Could you check a few things on this model? Use its own coordinates, in mm. A direction names the side the tool comes from. Coordinates: 2 decimals unless noted, no trailing zeros. Loops run counter-clockwise (first coordinate to the right, second up) from the corner with the lowest first, then second, coordinate; pieces in that order, holes last. Notation, with made-up numbers: (58, -29) -> (63, -29) arc R26 cw to (63, 8) -> close; hole circle Ø1 at (65, 71). An arc over 180 degrees is marked (long way). One line per question, with ' | ' between items.
from build123d import *

# Parameters (mm, degrees)
F0_R     = 2
F0_R_2   = 5
F1_DEPTH = 12
F2_R     = 2
F3_DEPTH = 25
F4_R     = 4.99999


# Not quite as in the source:
# - a fillet or chamfer is up to 0.001 mm smaller than in the source, because OpenCascade refuses the exact size


with BuildPart() as f1:
    # F0 (on Top) → F1 (new body)
    with BuildSketch(Plane.XY):
        with BuildLine():
            Line((-35.0000017881, -70), (35.0000017881, -70))
            ThreePointArc((35.0000017881, -70), (42.0710696, -67.0710678119), (45.0000017881, -60))
            Line((45.0000017881, -60), (45.0000017881, 70))
            Line((45.0000017881, 70), (-45.0000017881, 70))
            Line((-45.0000017881, 70), (-45.0000017881, -60))
            ThreePointArc((-45.0000017881, -60), (-42.0710696, -67.0710678119), (-35.0000017881, -70))
        make_face()
        with Locations((0, -30)):
            Circle(F0_R, mode=Mode.SUBTRACT)
        with Locations((0, 30)):
            Circle(F0_R, mode=Mode.SUBTRACT)
        with Locations((-35.0000017881, 60)):
            Circle(F0_R_2, mode=Mode.SUBTRACT)
        with Locations((0, 60)):
            Circle(F0_R_2, mode=Mode.SUBTRACT)
        with Locations((35.0000017881, 60)):
            Circle(F0_R_2, mode=Mode.SUBTRACT)
    extrude(amount=F1_DEPTH)

    # F2 (on face) → F3 (cut)
    with BuildSketch(Plane(origin=(0, 70, 0), x_dir=(-1, 0, 0), z_dir=(0, 1, 0))):
        with Locations((0, 6)):
            Circle(F2_R)
        with Locations((35.0000017881, 6)):
            Circle(F2_R)
        with Locations((-35.0000017881, 6)):
            Circle(F2_R)
    extrude(amount=-F3_DEPTH, mode=Mode.SUBTRACT)

    # F4 (radius 5 in the source; OpenCascade refuses exactly that, so slightly less here)
    f4_edges = [f1.edges().sort_by_distance(p)[0] for p in [
        (45.000002, 5, 0),
    ]]
    fillet(f4_edges, radius=F4_R)


solid = f1.part
1) If we section it at C-C on y = 60: Give the number of separate pieces and of enclosed holes in the cut face, and give its area (3 significant figures).
Data:
separate pieces: 4 | enclosed holes: 0 | area: 709 mm²
2) I'm going to push a flat-ended pin straight in: pin 1 Ø1.2 at (x, z) = (34.5, 6) entering from +Y. Where does the tip first touch, or does it pass through?
Data:
pin 1: y = 45
3) If we section it at B-B on x = 0: Please give me the cut outline in (y, z), and give its area (3 significant figures).
Data:
outline: (-70, 5) arc R5 ccw to (-65, 0) -> (-32, 0) -> (-32, 12) -> (-70, 12) -> close; (-28, 0) -> (28, 0) -> (28, 12) -> (-28, 12) -> close; (32, 0) -> (55, 0) -> (55, 4) -> (45, 4) -> (45, 8) -> (55, 8) -> (55, 12) -> (32, 12) -> close; (65, 0) -> (70, 0) -> (70, 4) -> (65, 4) -> close; (65, 8) -> (70, 8) -> (70, 12) -> (65, 12) -> close | area: 1,400 mm²
4) I need wall thicknesses on line 1 along X through (y, z) = (67.2, 6); line 2 along Z through (x, y) = (0, 49); line 3 along X through (y, z) = (-29, 11.75). Which ranges of each line are inside material? Lowest first, please. Write a range as from..to.
Data:
line 1: -45..-37, -33..-2, 2..33, 37..45 | line 2: 0..4, 8..12 | line 3: -45..-1.73, 1.73..45
5) If we section it at A-A on y = -30: Please give me the cut outline in (x, z), and give its area (3 significant figures).
Data:
outline: (-45, 5) arc R5 ccw to (-40, 0) -> (-2, 0) -> (-2, 12) -> (-45, 12) -> close; (2, 0) -> (40, 0) arc R5 ccw to (45, 5) -> (45, 12) -> (2, 12) -> close | area: 1,020 mm²
6) On a 3-axis mill with a long thin cutter (end or side, diameter ignored), from which of +Z, -Z, +X, -X, +Y, -Y can I reach the whole of each face in a straight line? I mean faces 1 (the face through (0, 45, 6)), 2 (the face through (-42.15, -66.99, 8.45)). Say none if no direction works.
Data:
face 1: +Y | face 2: +Z, -Z, -X, -Y
7) If we section it at D-D on z = 1.5: Please give me the cut outline in (x, y).
Data:
outline: (-43.57, -60) arc R8.57 ccw to (-35, -68.57) -> (35, -68.57) arc R8.57 ccw to (43.57, -60) -> (43.57, 70) -> (-43.57, 70) -> close; hole circle Ø10 at (-35, 60); hole circle Ø10 at (0, 60); hole circle Ø4 at (0, -30); hole circle Ø4 at (0, 30); hole circle Ø10 at (35, 60)
8) We'd pull the mould along X, two halves only. Please class faces 3 (the face through (-43, 4, 1)), 4 (the face through (4.77, 61.5, 5.92)), 5 (the face through (1, 70, 3)): pulls with the +X half, pulls with the -X half, needs draft (parallel to the pull), parting line crosses it, or undercut.
Data:
face 3: pulls with the -X half | face 4: undercut | face 5: needs draft
